from build123d import *

# Parameters (mm, degrees)
BOSS_EXTRUDE1_DEPTH                       = 25.4
TAPPED_HOLE_FOR_1_4_20_HELICOIL1_D        = 6.7564
TAPPED_HOLE_FOR_1_4_20_HELICOIL1_DEPTH    = 20.5232
TAPPED_HOLE_FOR_1_4_20_HELICOIL1_TIP      = 2.029827343
F_33_64_0_51563_DIAMETER_HOLE1_AT_2_COUNT = 2
F_33_64_0_51563_DIAMETER_HOLE1_AT_2_PITCH = 50.8
F_33_64_0_51563_DIAMETER_HOLE1_AT_3_COUNT = 2
F_33_64_0_51563_DIAMETER_HOLE1_AT_3_PITCH = 50.8
F_11_0_191_DIAMETER_HOLE1_AT_2_COUNT      = 2
F_11_0_191_DIAMETER_HOLE1_AT_2_PITCH      = 50.8
F_11_0_191_DIAMETER_HOLE1_AT_3_COUNT      = 2
F_11_0_191_DIAMETER_HOLE1_AT_3_PITCH      = 50.8


with BuildPart() as part:
    # Sketch1 → Boss-Extrude1 (new body)
    with BuildSketch(Plane.XY):
        with BuildLine():
            Line((0, 0), (0, 12.7))
            Line((0, 12.7), (20.139487758, 12.7))
            ThreePointArc((20.139487758, 12.7), (24.999567349, 13.666729937), (29.119743879, 16.419743879))
            Line((29.119743879, 16.419743879), (59.780256121, 47.080256121))
            ThreePointArc((59.780256121, 47.080256121), (62.533270063, 51.200432651), (63.5, 56.060512242))
            Line((63.5, 56.060512242), (63.5, 152.4))
            Line((63.5, 152.4), (76.2, 152.4))
            Line((76.2, 152.4), (76.2, 0))
            Line((76.2, 0), (0, 0))
        make_face()
    extrude(amount=BOSS_EXTRUDE1_DEPTH)

    # Tapped Hole for 1/4-20 Helicoil1
    with Locations(Plane.XZ):
        with Locations((19.05, 12.7), (50.8, 12.7)):
            Hole(TAPPED_HOLE_FOR_1_4_20_HELICOIL1_D / 2, depth=TAPPED_HOLE_FOR_1_4_20_HELICOIL1_DEPTH)
            with Locations((0, 0, -(TAPPED_HOLE_FOR_1_4_20_HELICOIL1_DEPTH + TAPPED_HOLE_FOR_1_4_20_HELICOIL1_TIP / 2))):  # 118° drill point
                Cone(0, TAPPED_HOLE_FOR_1_4_20_HELICOIL1_D / 2, TAPPED_HOLE_FOR_1_4_20_HELICOIL1_TIP, mode=Mode.SUBTRACT)

    # Sketch5 → 33/64 (0.51563) Diameter Hole1 (revolve, cut)
    with BuildSketch(Plane(origin=(0, 86.106, 12.7), x_dir=(0, 0, 1), z_dir=(0, 1, 0))):
        Polygon((0, 0), (0, 76.2), (8.453501, 76.2), (6.548501, 74.295), (6.548501, 0), align=None)
    f_33_64_0_51563_diameter_hole1 = revolve(axis=Axis((-6.35, 86.106, 12.7), (1, 0, 0)), mode=Mode.SUBTRACT)

    # 33/64 (0.51563) Diameter Hole1 at 2: 33/64 (0.51563) Diameter Hole1 ×2
    with Locations(*[(0, i * F_33_64_0_51563_DIAMETER_HOLE1_AT_2_PITCH, 0) for i in range(1, F_33_64_0_51563_DIAMETER_HOLE1_AT_2_COUNT)]):
        add(f_33_64_0_51563_diameter_hole1, mode=Mode.SUBTRACT)

    # 33/64 (0.51563) Diameter Hole1 at 3: 33/64 (0.51563) Diameter Hole1 ×2
    with Locations(*[(0, -i * F_33_64_0_51563_DIAMETER_HOLE1_AT_3_PITCH, 0) for i in range(1, F_33_64_0_51563_DIAMETER_HOLE1_AT_3_COUNT)]):
        add(f_33_64_0_51563_diameter_hole1, mode=Mode.SUBTRACT)

    # Sketch7 → #11 (0.191) Diameter Hole1 (revolve, cut)
    with BuildSketch(Plane(origin=(69.85, 86.106, 25.4), x_dir=(0, -1, 0), z_dir=(1, 0, 0))):
        Polygon((0, 0), (0, 25.4), (3.175, 25.4), (2.4257, 24.6507), (2.4257, 0.7493), (3.175, 0), align=None)
    f_11_0_191_diameter_hole1 = revolve(axis=Axis((69.85, 86.106, 31.75), (0, 0, -1)), mode=Mode.SUBTRACT)

    # #11 (0.191) Diameter Hole1 at 2: #11 (0.191) Diameter Hole1 ×2
    with Locations(*[(0, i * F_11_0_191_DIAMETER_HOLE1_AT_2_PITCH, 0) for i in range(1, F_11_0_191_DIAMETER_HOLE1_AT_2_COUNT)]):
        add(f_11_0_191_diameter_hole1, mode=Mode.SUBTRACT)

    # #11 (0.191) Diameter Hole1 at 3: #11 (0.191) Diameter Hole1 ×2
    with Locations(*[(0, -i * F_11_0_191_DIAMETER_HOLE1_AT_3_PITCH, 0) for i in range(1, F_11_0_191_DIAMETER_HOLE1_AT_3_COUNT)]):
        add(f_11_0_191_diameter_hole1, mode=Mode.SUBTRACT)


solid = part.part
Input: part model. Units: mm. Frame: model coordinates. A direction names the side the tool comes from. Give positions to 0.01 mm unless a question says otherwise; leave off trailing zeros. Write each loop counter-clockwise with the first axis right and the second up, starting at its lowest first coordinate (ties: lowest second). Pieces come first, ordered by that corner, then holes. Notation, with made-up numbers: M 40,-6 L 79,-6 A22 ccw 79,13 Z; hole C -9,49.25 d2. An arc over 180 degrees is marked long. Use one line per item in the form item = value.
1. Reachability of faces 1 (the face through (67.445, 86.422, 21.758)), 2 (the face through (10, 12.7, 13)), 3 (the face through (47.578, 10.405, 13.715)) from +Z, -Z, +X, -X, +Y, -Y: full face, straight path, thin tool, end or side. Return the list, or none.
Outcome:
face_1 = +Z, -Z
face_2 = +Z, -Z, -X, +Y
face_3 = -Y
2. Cut plane B-B on y = 127. Return loops of the section in (x, z).
Outcome:
outline = M 63.5,0 L 76.2,0 L 76.2,25.4 L 63.5,25.4 Z
3. Cut plane A-A on x = 69.85. State how many separate pieces and enclosed holes the cut face has, and give its area (3 significant figures).
Outcome:
separate_pieces = 4
enclosed_holes = 0
area = 3,280 mm²
4. Ray query, L1, parallel to Y at x = 69.85, z = 4; L2, parallel to Y at x = 69.5, z = 12.7; L3, parallel to X at y = 11, z = 12.7. Return the intervals inside material, ascending.
Outcome:
L1 = 0 to 32.88, 37.73 to 83.68, 88.53 to 134.48, 139.33 to 152.4
L2 = 0 to 28.76, 41.85 to 79.56, 92.65 to 130.36, 143.45 to 152.4
L3 = 0 to 15.67, 22.43 to 47.42, 54.18 to 76.2
5. Mould query, pull axis X, two halves, no side actions, for faces 4 (the face through (67.445, 137.222, 21.758)), 5 (the face through (76.2, 77, 13)), 6 (the face through (69.74, 88.53, 3.72)), 7 (the face through (70, 152.4, 13)). Classes: released by +X, released by -X, zero draft, split by the parting line, or undercut.
Outcome:
face_4 = undercut
face_5 = released by +X
face_6 = undercut
face_7 = zero draft
6. First-contact query: P1, Ø5.5, axis at x = 69.85, y = 35.306, coming from the +Z side (3 decimals); P2, Ø8, axis at x = 69.85, y = 86.106, coming from the -Z side; P3, Ø8, axis at y = 136.906, z = 12.7, coming from the -X side; P4, Ø12, axis at y = 41, z = 21.5, coming from the -X side. Flat tips, straight axial feed; report the tip coordinate or a pass-through.
Outcome:
P1 = 24.975
P2 = 0
P3 = through
P4 = 47.7
7. Cut plane C-C on y = 52. Return loops of the section in (x, z), and give its area (3 significant figures).
Outcome:
outline = M 62.83,0 L 76.2,0 L 76.2,25.4 L 62.83,25.4 Z
area = 340 mm²
